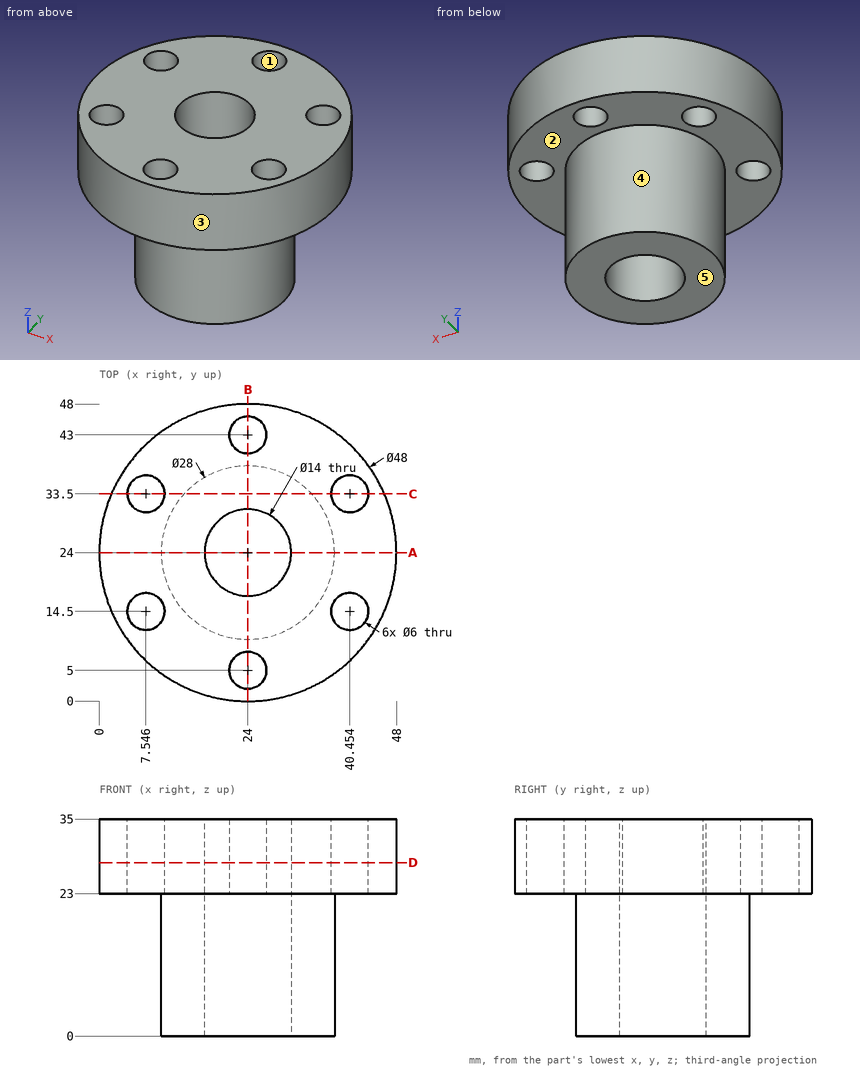
Geometry check sheet. Reference: drawing and pictorial views, mm from the part's lowest x, y, z. A direction names the side the tool comes from. Coordinates: 2 decimals unless noted, no trailing zeros. Loops run counter-clockwise (first coordinate to the right, second up) from the corner with the lowest first, then second, coordinate; pieces in that order, holes last. Notation, with made-up numbers: (62, 15.25) -> (71, 15.25) arc R28 cw to (71, 44.25) -> close; hole circle Ø2 at (-1.75, -16). An arc over 180 degrees is marked (long way). Put each result on its own line as item: value.
1) Cross-section at C-C on y = 33.5. Record the boundary of the cut face in (x, z) (1 decimal).
Result set:
outline: (2, 23) -> (4.5, 23) -> (4.5, 35) -> (2, 35) -> close; (10.5, 23) -> (13.7, 23) -> (13.7, 0) -> (34.3, 0) -> (34.3, 23) -> (37.5, 23) -> (37.5, 35) -> (10.5, 35) -> close; (43.5, 23) -> (46, 23) -> (46, 35) -> (43.5, 35) -> close
2) Cross-section at B-B on x = 24. Record the boundary of the cut face in (y, z).
Result set:
outline: (0, 23) -> (2, 23) -> (2, 35) -> (0, 35) -> close; (8, 23) -> (10, 23) -> (10, 0) -> (17, 0) -> (17, 35) -> (8, 35) -> close; (31, 0) -> (38, 0) -> (38, 23) -> (40, 23) -> (40, 35) -> (31, 35) -> close; (46, 23) -> (48, 23) -> (48, 35) -> (46, 35) -> close
3) Release check for a two-part mould opening along X. For the marked faces 1, 2 and 3 record: released by +X, released by -X, zero draft, split by the parting line, or undercut.
Result set:
face 1: undercut
face 2: zero draft
face 3: split by the parting line
4) Cross-section at D-D on z = 28. Record the boundary of the cut face in (x, y) (1 decimal), plus the area to 3 significant figures.
Result set:
outline: circle Ø48 at (24, 24); hole circle Ø6 at (7.5, 14.5); hole circle Ø6 at (7.5, 33.5); hole circle Ø14 at (24, 24); hole circle Ø6 at (24, 5); hole circle Ø6 at (24, 43); hole circle Ø6 at (40.5, 14.5); hole circle Ø6 at (40.5, 33.5)
area: 1,490 mm^2
5) Thickness scan on line 1 (Y direction, x = 21.5, z = 23.5) (1 decimal); line 2 (Z direction, x = 33.5, y = 12.5); line 3 (Y direction, x = 9, z = 30) (1 decimal). Record the ranges inside material, lowest first.
Result set:
line 1: y = 0.1 to 3.3, 6.7 to 17.5, 30.5 to 41.3, 44.7 to 47.9
line 2: z = 23 to 35
line 3: y = 5.3 to 11.9, 17.1 to 30.9, 36.1 to 42.7
6) Gauge pin test, flat ends, axial feed: pin 1 Ø5 at (x, y) = (24, 43) entering from -Z; pin 2 Ø1 at (x, z) = (13.5, 28) entering from -Y; pin 3 Ø8 at (y, z) = (17.5, 10.5) entering from -X (1 decimal); pin 4 Ø1.5 at (y, z) = (26.5, 7.5) entering from -X. Record the tip position at first contact, or that the pin passes through.
Result set:
pin 1: passes through
pin 2: stops at y = 2.18
pin 3: stops at x = 10.2
pin 4: stops at x = 10.11
7) Tool access check on the marked faces 4 and 5. Record the directions out of +Z, -Z, +X, -X, +Y, -Y that give a thin tool (end or side, any length) a straight path to the whole face; none if there is none.
Result set:
face 4: -Z
face 5: -Z, +X, -X, +Y, -Y
8) Cross-section at A-A on y = 24. Record the boundary of the cut face in (x, z), plus the area to 3 significant figures.
Result set:
outline: (0, 23) -> (10, 23) -> (10, 0) -> (17, 0) -> (17, 35) -> (0, 35) -> close; (31, 0) -> (38, 0) -> (38, 23) -> (48, 23) -> (48, 35) -> (31, 35) -> close
area: 730 mm^2
